```python
from build123d import *

# Parameters (mm, degrees)
F0_W     = 25.4
F0_H     = 1828.8
F1_DEPTH = 25.4
F2_W     = 25.4
F2_H     = 20.32
F3_DEPTH = 25.4
F4_W     = 50.8
F4_H     = 20.32
F5_DEPTH = 25.4
F6_R     = 3.175
F7_DEPTH = 50.8


with BuildPart() as f1:
    # F0 (on Top) → F1 (new body)
    with BuildSketch(Plane.XY):
        Rectangle(F0_W, F0_H)
    extrude(amount=F1_DEPTH)

    # F2 (on face) → F3 (cut)
    with BuildSketch(Plane(origin=(-12.7, 0, 0), x_dir=(0, -1, 0), z_dir=(-1, 0, 0))):
        with Locations((-927.1, 12.7)):
            Rectangle(F2_W, F2_H)
        with Locations((-901.7, 12.7)):
            Rectangle(F2_W, F2_H)
    extrude(amount=-F3_DEPTH, mode=Mode.SUBTRACT)

    # F4 (on face) → F5 (cut)
    with BuildSketch(Plane(origin=(-12.7, 0, 0), x_dir=(0, -1, 0), z_dir=(-1, 0, 0))):
        with Locations((914.4, 12.7)):
            Rectangle(F4_W, F4_H)
    extrude(amount=-F5_DEPTH, mode=Mode.SUBTRACT)

    # F6 (on face) → F7 (cut)
    with BuildSketch(Plane.XY.offset(25.4)):
        with Locations((0, 904.875)):
            Circle(F6_R)
        with Locations((0, -904.875)):
            Circle(F6_R)
    extrude(amount=-F7_DEPTH, mode=Mode.SUBTRACT)


solid = f1.part
```
Build history of the part. All positions in model axes, mm. Round coordinates to 2 decimals unless told otherwise and drop trailing zeros. Write each loop counter-clockwise with the first axis right and the second up, starting at its lowest first coordinate (ties: lowest second). Pieces come first, ordered by that corner, then holes. Notation, with made-up numbers: (83.25, 25.25) -> (112.25, 25.25) arc R25 cw to (112.25, 56.25) -> close; hole circle Ø11 at (-26, 22.5). An arc over 180 degrees is marked (long way). Put each result on its own line as item: value.
Item 1: Flat gauge pins, fed straight in: P1, Ø4, axis at x = 9, z = 16.5, coming from the -Y side; P2, Ø8, axis at x = -3.5, z = 10, coming from the +Y side. Where does each tip first touch, or does it go through?
Here are the results:
P1: stops at y = -889
P2: stops at y = 889
Item 2: Slice it at B-B, the plane z = 12.5. Give the cut face in (x, y), plus the area to 3 significant figures.
Here are the results:
outline: (-12.7, -889) -> (12.7, -889) -> (12.7, 889) -> (-12.7, 889) -> close
area: 45,200 mm^2
Item 3: Slice it at A-A, the plane x = -7. Give the cut face in (y, z).
Here are the results:
outline: (-914.4, 0) -> (914.4, 0) -> (914.4, 2.54) -> (889, 2.54) -> (889, 22.86) -> (914.4, 22.86) -> (914.4, 25.4) -> (-914.4, 25.4) -> (-914.4, 22.86) -> (-889, 22.86) -> (-889, 2.54) -> (-914.4, 2.54) -> close
Item 4: Wall check: probe 1 along Y at (x, z) = (0, 24.25); probe 2 along Y at (x, z) = (-2.5, 23.75); probe 3 along Y at (x, z) = (-5.75, 18). Give the ranges that are in metal, low to high. Write a range as from..to.
Here are the results:
probe 1: y = -914.4..-908.05, -901.7..901.7, 908.05..914.4
probe 2: y = -914.4..-906.83, -902.92..902.92, 906.83..914.4
probe 3: y = -889..889
